Design review of the part built by this model. Coordinates are the model's own, in mm. Coordinates: 2 decimals unless noted, no trailing zeros. Order: outer loops, then holes, each group sorted by start corner. A loop starts at its lowest first (then second) coordinate and runs counter-clockwise, first axis right, second up. Notation, with made-up numbers: M 80,-40 L 139,-40 A17 cw 139,-9 Z; hole C -11.75,-31 d11. An arc over 180 degrees is marked long. Answer in a Markdown table with one row per item.
from build123d import *

# Parameters (mm, degrees)
EXTRUDE_1_DEPTH     = 3
SKETCH_7_R          = 11
CUT_EXTRUDE_4_DEPTH = 116.299609713
SKETCH_9_R          = 0.8
SKETCH_9_R_2        = 0.825279091
CUT_EXTRUDE_5_DEPTH = 113.379793517


with BuildPart() as part:
    # 草图4 → 凸台-拉伸1 (new body)
    with BuildSketch(Plane(origin=(0, 0, 0), x_dir=(1, 0, 0), z_dir=(0, 1, 0))):
        Polygon((-47, 82), (47, 82), (81, 0), (47, -82), (-47, -82), (-81, 0), align=None)
    extrude(amount=EXTRUDE_1_DEPTH)

    # 草图7 → 切除-拉伸4 (cut, through all)
    with BuildSketch(Plane(origin=(0, 3, 0), x_dir=(1, 0, 0), z_dir=(0, 1, 0))):
        with Locations((-81, 0)):
            Circle(SKETCH_7_R)
        with Locations((-47, 82)):
            Circle(SKETCH_7_R)
        with Locations((47, 82)):
            Circle(SKETCH_7_R)
        with Locations((81, 0)):
            Circle(SKETCH_7_R)
        with Locations((47, -82)):
            Circle(SKETCH_7_R)
        with Locations((-47, -82)):
            Circle(SKETCH_7_R)
    extrude(amount=-CUT_EXTRUDE_4_DEPTH, mode=Mode.SUBTRACT)

    # 草图9 → 切除-拉伸5 (cut, through all)
    with BuildSketch(Plane(origin=(0, 3, 0), x_dir=(1, 0, 0), z_dir=(0, 1, 0))):
        with Locations(Location((-53.5, 0, 0), (0, 0, 270))):
            Circle(SKETCH_9_R)
        with Locations(Location((-60.5, 7, 0), (0, 0, 270))):
            Circle(SKETCH_9_R_2)
        with Locations(Location((-60.5, -7, 0), (0, 0, 90))):
            Circle(SKETCH_9_R_2)
        with Locations(Location((-27.554563517, -62.554563517, 0), (0, 0, 270))):
            Circle(SKETCH_9_R)
        with Locations(Location((-37.454058454, -62.554563517, 0), (0, 0, 270))):
            Circle(SKETCH_9_R)
        with Locations(Location((-27.554563517, -72.454058454, 0), (0, 0, 90))):
            Circle(SKETCH_9_R)
        with Locations(Location((-27.554563517, 62.554563517, 0), (0, 0, 270))):
            Circle(SKETCH_9_R)
        with Locations(Location((-27.554563517, 72.454058454, 0), (0, 0, 270))):
            Circle(SKETCH_9_R)
        with Locations(Location((-37.454058454, 62.554563517, 0), (0, 0, 90))):
            Circle(SKETCH_9_R)
    cut_extrude_5 = extrude(amount=-CUT_EXTRUDE_5_DEPTH, mode=Mode.SUBTRACT)

    # 镜向2: 切除-拉伸5 across plane
    add(cut_extrude_5.mirror(Plane(origin=(0, 0, 0), x_dir=(0, 0, 1), z_dir=(1, 0, 0))), mode=Mode.SUBTRACT)


solid = part.part
(1) Add section B-B, the plane z = -45. Give the boundary of the cut face in (x, y), and give its area (3 significant figures).
Return value:
| item | result |
|---|---|
| outline | M -62.34,0 L 62.34,0 L 62.34,3 L -62.34,3 Z |
| area | 374 mm2 |
(2) Draft analysis for pull direction Z (two halves, no side actions). For faces 1 (the flat face through (-64, 1, 41)), 2 (the cylindrical face through (-70, 2, 0)), 3 (the cylindrical face through (40.765, 1.521, -72.938)), state which applies: pulls with the +Z half, pulls with the -Z half, needs draft (parallel to the pull), parting line crosses it, or undercut.
Return value:
| item | result |
|---|---|
| face 1 | pulls with the +Z half |
| face 2 | undercut |
| face 3 | pulls with the -Z half |
(3) Insertion check: pin 1 Ø2 at (x, z) = (27.55, -72.45) entering from +Y; pin 2 Ø1 at (x, z) = (-60.5, -7) entering from +Y. Each pin has a flat end and moves straight along its axis. Give the tip position at first contact, or say it passes through.
Return value:
| item | result |
|---|---|
| pin 1 | stops at y = 3 |
| pin 2 | passes through |
(4) Add section A-A, the plane y = 1.2. Give the number of separate pieces and of enclosed holes in the cut face, and give its area (3 significant figures).
Return value:
| item | result |
|---|---|
| separate pieces | 1 |
| enclosed holes | 18 |
| area | 20,200 mm2 |
(5) Add section C-C, the plane x = -65.5. Give the boundary of the cut face in (y, z).
Return value:
| item | result |
|---|---|
| outline | M 0,-37.38 L 3,-37.38 L 3,37.38 L 0,37.38 Z |
(6) For line 1 along X through (y, z) = (2.45, -7); line 2 along Z through (x, y) = (-60.5, 1.15); line 3 along X through (y, z) = (2.85, 4.5), list the stretches that pass through material, from the lowest coordinate up. Write a range as from..to.
Return value:
| item | result |
|---|---|
| line 1 | x = -72.51..-61.33, -59.67..59.67, 61.33..72.51 |
| line 2 | z = -49.44..-7.83, -6.17..6.17, 7.83..49.44 |
| line 3 | x = -70.96..70.96 |
